from build123d import *

# Parameters (mm, degrees)
F0_R     = 63.5
F1_DEPTH = 25.4
F4_R     = 3.175
F5_DEPTH = 12.7
F6_R     = 3.175
F7_DEPTH = 12.7


with BuildPart() as f1:
    # F0 (on Front) → F1 (new body)
    with BuildSketch(Plane.XZ):
        Circle(F0_R)
    extrude(amount=F1_DEPTH)

    # F4 (on face) → F5 (cut)
    with BuildSketch(Plane.XZ.offset(25.4)):
        Circle(F4_R)
    extrude(amount=-F5_DEPTH, mode=Mode.SUBTRACT)

    # F6 (on face) → F7 (cut)
    with BuildSketch(Plane(origin=(0, 0, 0), x_dir=(-1, 0, 0), z_dir=(0, 1, 0))):
        with Locations((-12.7, 0)):
            Circle(F6_R)
        with Locations((12.7, 0)):
            Circle(F6_R)
    extrude(amount=-F7_DEPTH, mode=Mode.SUBTRACT)


solid = f1.part
Work out the finished part from the listing and answer in its coordinate system (mm). A direction names the side the tool comes from. Give positions to 0.01 mm unless a question says otherwise; leave off trailing zeros. Loops run counter-clockwise (first coordinate to the right, second up) from the corner with the lowest first, then second, coordinate; pieces in that order, holes last. Notation, with made-up numbers: (7.5, 28) -> (43.5, 28) arc R20 cw to (43.5, 62) -> close; hole circle Ø4 at (7, -11). An arc over 180 degrees is marked (long way). Use a Markdown table: item, result. Add a question column.
1) Which of the six approach directions +Z, -Z, +X, -X, +Y, -Y give full straight-line access (tool end or side, diameter ignored) to faces 5 (the flat face through (13, -25.4, 1)), 6 (the cylindrical face through (-9.53, -6.26, 0.14)), 7 (the flat face through (0, -12.7, 0))?
2) Each of these flat-tipped pins is pushed along its axis until it touches: P1, Ø8, axis at y = -9.5, z = 48.5, coming from the -X side; P2, Ø8, axis at y = -21.5, z = 16.5, coming from the -X side; P3, Ø4, axis at y = -7.5, z = 12.5, coming from the +X side. Where does it stop, or does it pass through?
3) The part is cut by section D-D, the plane y = -8.75. Determine the outline of the cut face in (x, z) (3 decimals).
4) For a pull along X with two mould halves and no side action, classify faces 1 (the flat face through (-1, 0, 1)), 2 (the cylindrical face through (-13.77, -12.52, -61.99)), 3 (the cylindrical face through (9.67, -6.26, 0.95)), 4 (the flat face through (13, -12.7, 0)) as +X half, -X half, draft (parallel to the pull), parting line (faces both ways), or undercut.
5) The part is cut by section B-B, the plane z = 0. Determine the outline of the cut face in (x, y) (3 decimals), plus the area to 3 significant figures.
6) The part is cut by section C-C, the plane y = -20.5. Determine the outline of the cut face in (x, z) (3 decimals), plus the area to 3 significant figures.
7) Consider line 1 along Z through (x, y) = (0, -22.75) (3 decimals); line 2 along Z through (x, y) = (12.7, -4.75) (3 decimals); line 3 along X through (y, z) = (-21.5, 1). Determine where each line is inside the solid, lowest interval first.
8) The part is cut by section A-A, the plane x = 0. Determine the outline of the cut face in (y, z) (3 decimals).
Reported:
| question | item | result |
|---|---|---|
| 1 | face 5 | +Z, -Z, +X, -X, -Y |
| 1 | face 6 | +Y |
| 1 | face 7 | -Y |
| 2 | P1 | stops at x = -45.3 |
| 2 | P2 | stops at x = -62.26 |
| 2 | P3 | stops at x = 62.63 |
| 3 | outline | circle Ø127 at (0, 0); hole circle Ø6.35 at (-12.7, 0); hole circle Ø6.35 at (12.7, 0) |
| 4 | face 1 | draft |
| 4 | face 2 | parting line |
| 4 | face 3 | undercut |
| 4 | face 4 | undercut |
| 5 | outline | (-63.5, -25.4) -> (-3.175, -25.4) -> (-3.175, -12.7) -> (3.175, -12.7) -> (3.175, -25.4) -> (63.5, -25.4) -> (63.5, 0) -> (15.875, 0) -> (15.875, -12.7) -> (9.525, -12.7) -> (9.525, 0) -> (-9.525, 0) -> (-9.525, -12.7) -> (-15.875, -12.7) -> (-15.875, 0) -> (-63.5, 0) -> close |
| 5 | area | 2,980 mm^2 |
| 6 | outline | circle Ø127 at (0, 0); hole circle Ø6.35 at (0, 0) |
| 6 | area | 12,600 mm^2 |
| 7 | line 1 | z = -63.5 to -3.175, 3.175 to 63.5 |
| 7 | line 2 | z = -62.217 to -3.175, 3.175 to 62.217 |
| 7 | line 3 | x = -63.49 to -3.01, 3.01 to 63.49 |
| 8 | outline | (-25.4, -63.5) -> (0, -63.5) -> (0, 63.5) -> (-25.4, 63.5) -> (-25.4, 3.175) -> (-12.7, 3.175) -> (-12.7, -3.175) -> (-25.4, -3.175) -> close |
